```python
from build123d import *

# Parameters (mm, degrees)
SKETCH1_W                   = 25.4
SKETCH1_H                   = 15.875
BOSS_EXTRUDE1_DEPTH         = 7.9375
CUT_EXTRUDE1_REACH          = 27.4
SKETCH2_W                   = 3.81
SKETCH2_H                   = 3.8735
F_1_4_20_TAPPED_HOLE1_D     = 5.1054
F_1_4_20_TAPPED_HOLE1_DEPTH = 16.51
F_1_4_20_TAPPED_HOLE1_TIP   = 1.533816902


with BuildPart() as part:
    # Sketch1 → Boss-Extrude1 (new body)
    with BuildSketch(Plane.XY):
        Rectangle(SKETCH1_W, SKETCH1_H)
    extrude(amount=BOSS_EXTRUDE1_DEPTH)

    # Sketch2 → Cut-Extrude1 (cut, up to next)
    with BuildSketch(Plane(origin=(12.7, 0, 0), x_dir=(0, 0, -1), z_dir=(1, 0, 0)), mode=Mode.PRIVATE) as cut_extrude1_sk1:
        with Locations((-6.0325, 6.00075)):
            Rectangle(SKETCH2_W, SKETCH2_H)
    cut_extrude1_tool1 = extrude(cut_extrude1_sk1.sketch, amount=-CUT_EXTRUDE1_REACH, mode=Mode.PRIVATE) & part.part
    add(cut_extrude1_tool1.solids().sort_by_distance((12.7, 6.00075, 6.0325))[0], mode=Mode.SUBTRACT)
    # Sketch2 → Cut-Extrude1 (cut, up to next)
    with BuildSketch(Plane(origin=(12.7, 0, 0), x_dir=(0, 0, -1), z_dir=(1, 0, 0)), mode=Mode.PRIVATE) as cut_extrude1_sk2:
        with Locations((-6.0325, -6.00075)):
            Rectangle(SKETCH2_W, SKETCH2_H)
    cut_extrude1_tool2 = extrude(cut_extrude1_sk2.sketch, amount=-CUT_EXTRUDE1_REACH, mode=Mode.PRIVATE) & part.part
    add(cut_extrude1_tool2.solids().sort_by_distance((12.7, -6.00075, 6.0325))[0], mode=Mode.SUBTRACT)

    # 1/4-20 Tapped Hole1
    with Locations(Plane.XY.offset(7.9375)):
        with Locations((0, 0)):
            Hole(F_1_4_20_TAPPED_HOLE1_D / 2, depth=F_1_4_20_TAPPED_HOLE1_DEPTH)
            with Locations((0, 0, -(F_1_4_20_TAPPED_HOLE1_DEPTH + F_1_4_20_TAPPED_HOLE1_TIP / 2))):  # 118° drill point
                Cone(0, F_1_4_20_TAPPED_HOLE1_D / 2, F_1_4_20_TAPPED_HOLE1_TIP, mode=Mode.SUBTRACT)


solid = part.part
```
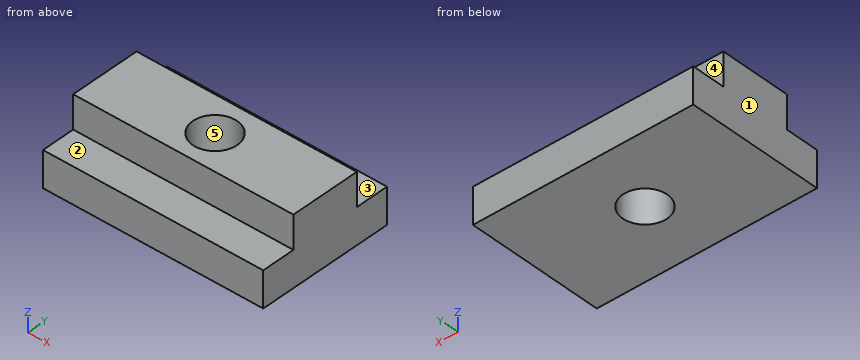
Check sheet for the modelled part. Datum: model origin and axes. Units: mm. Face numbers are marked on the shaded views. A direction names the side the tool comes from. Give positions to 0.01 mm unless a question says otherwise; leave off trailing zeros. Order: outer loops, then holes, each group sorted by start corner. A loop starts at its lowest first (then second) coordinate and runs counter-clockwise, first axis right, second up. Notation, with made-up numbers: M 6.5,85.25 L 58.5,85.25 A11 ccw 58.5,105.25 Z; hole C 39.25,88 d9. An arc over 180 degrees is marked long. Answer in a Markdown table with one row per item. Add a question column.
Q1. Sectioned sample at C-C, the plane z = 2.75. Record the boundary of the cut face in (x, y).
Q2. Thickness scan on L1, parallel to Z at x = 11, y = 4.75; L2, parallel to Y at x = -1, z = 3.75; L3, parallel to X at y = -1.75, z = 3.5. Record the ranges inside material, lowest first.
Q3. Sectioned sample at B-B, the plane x = 0. Record the boundary of the cut face in (y, z).
Q4. Gauge pin test, flat ends, axial feed: pin 1 Ø3 at (x, y) = (-5.5, 6.5) entering from +Z; pin 2 Ø1.1 at (x, z) = (-5.5, 7) entering from +Y; pin 3 Ø4 at (x, y) = (0, 0) entering from -Z; pin 4 Ø1 at (x, z) = (-2, 5) entering from -Y. Record the tip position at first contact, or that the pin passes through.
Q5. Sectioned sample at D-D, the plane x = 10.5. Record the boundary of the cut face in (y, z).
Q6. Release check for a two-part mould opening along Y. For the marked faces 3, 4 and 5 record: released by +Y, released by -Y, zero draft, split by the parting line, or undercut.
Q7. Sectioned sample at A-A, the plane y = 0. Record the boundary of the cut face in (x, z).
Q8. Access from +Z, -Z, +X, -X, +Y, -Y to the whole of each face (thin tool, end or side, straight path). Record for the marked faces 1 and 2.
Verdict:
| question | item | result |
|---|---|---|
| 1 | outline | M -12.7,-7.94 L 12.7,-7.94 L 12.7,7.94 L -12.7,7.94 Z; hole C 0,0 d5.11 |
| 2 | L1 | 0 to 4.13 |
| 2 | L2 | -7.94 to -2.35, 2.35 to 7.94 |
| 2 | L3 | -12.7 to -1.86, 1.86 to 12.7 |
| 3 | outline | M -7.94,0 L -2.55,0 L -2.55,7.94 L -4.06,7.94 L -4.06,4.13 L -7.94,4.13 Z; M 2.55,0 L 7.94,0 L 7.94,4.13 L 4.06,4.13 L 4.06,7.94 L 2.55,7.94 Z |
| 4 | pin 1 | z = 4.13 |
| 4 | pin 2 | y = 4.06 |
| 4 | pin 3 | through |
| 4 | pin 4 | y = -4.06 |
| 5 | outline | M -7.94,0 L 7.94,0 L 7.94,4.13 L 4.06,4.13 L 4.06,7.94 L -4.06,7.94 L -4.06,4.13 L -7.94,4.13 Z |
| 6 | face 3 | zero draft |
| 6 | face 4 | released by +Y |
| 6 | face 5 | undercut |
| 7 | outline | M -12.7,0 L -2.55,0 L -2.55,7.94 L -12.7,7.94 Z; M 2.55,0 L 12.7,0 L 12.7,7.94 L 2.55,7.94 Z |
| 8 | face 1 | +Z, -Z, -X, +Y, -Y |
| 8 | face 2 | +Z, +X, -X, -Y |
